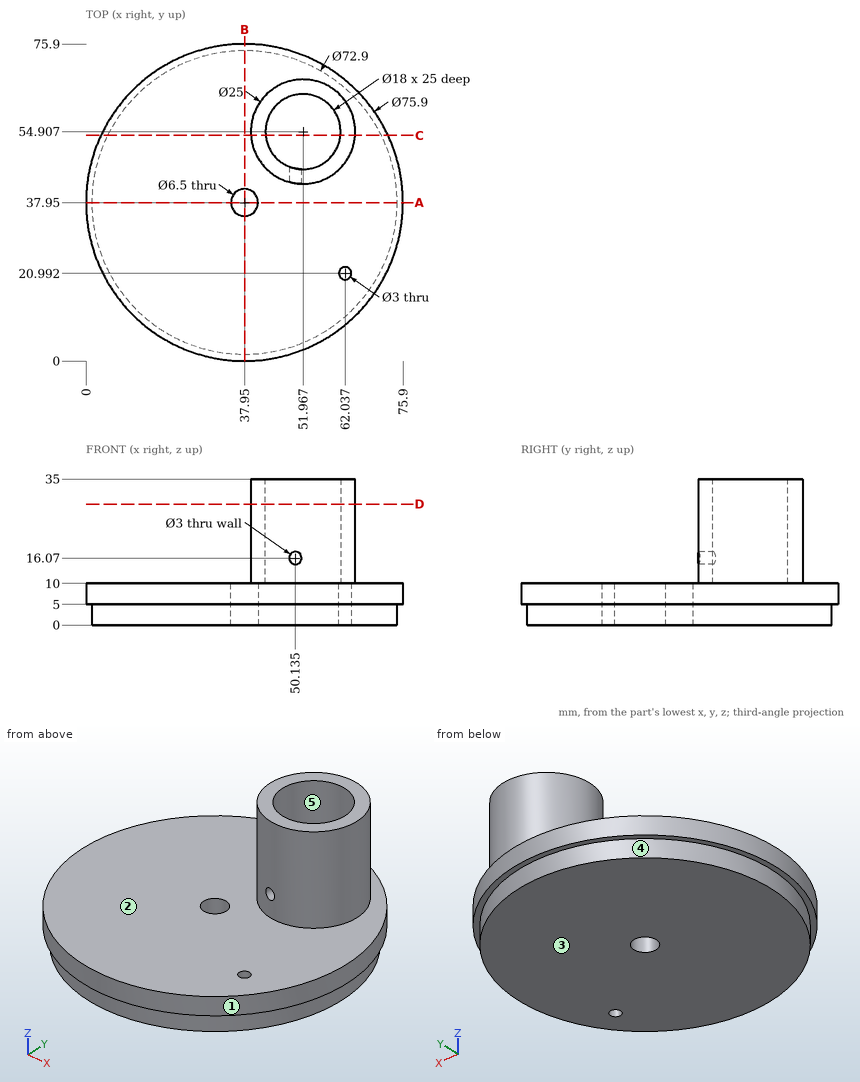
Can you work these out from the drawing? Everything is in mm from the part's minimum corner. A direction names the side the tool comes from. Coordinates: 2 decimals unless noted, no trailing zeros. Loops run counter-clockwise (first coordinate to the right, second up) from the corner with the lowest first, then second, coordinate; pieces in that order, holes last.
1) Imagine slicing it at A-A (y = 37.95). List the corners of the cut face in (x, z) for me.
Reported:
outline: (0, 5) - (1.5, 5) - (1.5, 0) - (34.7, 0) - (34.7, 10) - (0, 10) - close; (41.2, 0) - (74.4, 0) - (74.4, 5) - (75.9, 5) - (75.9, 10) - (41.2, 10) - close
2) Thinking about a two-plate mould opening in Z: for the marked faces 1, 2 and 3, which applies, released by +Z, released by -Z, zero draft, split by the parting line, or undercut?
Reported:
face 1: zero draft
face 2: released by +Z
face 3: released by -Z
3) Imagine slicing it at C-C (y = 54). List the corners of the cut face in (x, z) for me, and give its area (3 significant figures).
Reported:
outline: (3.56, 5) - (5.22, 5) - (5.22, 0) - (70.68, 0) - (70.68, 5) - (72.34, 5) - (72.34, 10) - (64.43, 10) - (64.43, 35) - (60.92, 35) - (60.92, 10) - (43.01, 10) - (43.01, 35) - (39.5, 35) - (39.5, 10) - (3.56, 10) - close
area: 847 mm2
4) Which directions (+Z, -Z, +X, -X, +Y, -Y) give clear straight access to the entire face, cutting with the end or side of a thin tool? Please do the marked faces 4 and 5.
Reported:
face 4: -Z
face 5: +Z
5) Will these pins go through, and if not, where does the flat tip stop? pin 1 Ø3 at (x, z) = (42, 16) entering from +Y; pin 2 Ø5 at (y, z) = (66, 15.5) entering from -X; pin 3 Ø6 at (y, z) = (53.5, 17.5) entering from +X.
Reported:
pin 1: stops at y = 64.1
pin 2: stops at x = 42.89
pin 3: stops at x = 64.47
6) Imagine slicing it at D-D (z = 29). List the corners of the cut face in (x, y) for me.
Reported:
outline: circle Ø25 at (51.97, 54.91); hole circle Ø18 at (51.97, 54.91)
7) Please list where these lines run through material, in increasing order: line 1 along Z through (x, y) = (46, 42); line 2 along Y through (x, z) = (53, 16); line 3 along X through (y, z) = (61, 11) (1 decimal).
Reported:
line 1: z = 0 to 10
line 2: y = 42.45 to 45.97, 63.85 to 67.36
line 3: x = 41.1 to 45.3, 58.6 to 62.9
